Input: part model. Units: mm. Frame: model coordinates. A direction names the side the tool comes from. Coordinates: 2 decimals unless noted, no trailing zeros. Order: outer loops, then holes, each group sorted by start corner. A loop starts at its lowest first (then second) coordinate and runs counter-clockwise, first axis right, second up. Notation, with made-up numbers: M 86.25,63.25 L 137.25,63.25 A15 ccw 137.25,84.25 Z; hole C 66.5,-35 d6. An arc over 180 degrees is marked long. Answer in a Markdown table with one row per item.
from build123d import *

# Parameters (mm, degrees)
CROQUIS1_R              = 55
SALIENTE_EXTRUIR1_DEPTH = 5
CROQUIS2_R              = 1.75
CROQUIS2_R_2            = 32.5
CORTAR_EXTRUIR1_DEPTH   = 78.942286341


with BuildPart() as part:
    # Croquis1 → Saliente-Extruir1 (new body)
    with BuildSketch(Plane.XY):
        Circle(CROQUIS1_R)
    extrude(amount=SALIENTE_EXTRUIR1_DEPTH)

    # Croquis2 → Cortar-Extruir1 (cut, through all)
    with BuildSketch(Plane.XY.offset(5)):
        with Locations((0, 50)):
            Circle(CROQUIS2_R)
        with Locations((43.301270189, 25)):
            Circle(CROQUIS2_R)
        with Locations((43.301270189, -25)):
            Circle(CROQUIS2_R)
        with Locations((0, -50)):
            Circle(CROQUIS2_R)
        with Locations((-43.301270189, -25)):
            Circle(CROQUIS2_R)
        with Locations((-43.301270189, 25)):
            Circle(CROQUIS2_R)
        with Locations((0.001598992, 0.000923179)):
            Circle(CROQUIS2_R_2)
        Polygon((-21.158630785, 50.828665682), (-16.028328636, 36.733276371), (-11.329865532, 38.443377087), (-16.460167682, 52.538766399), align=None)
        Polygon((16.028328636, 36.733276371), (11.329865532, 38.443377087), (16.460167682, 52.538766399), (21.158630785, 50.828665682), align=None)
        Polygon((54.598231114, -7.090421072), (39.826114819, -4.485698407), (38.957873931, -9.409737172), (53.729990226, -12.014459837), align=None)
        Polygon((27.628008399, -29.033639916), (37.269822544, -40.524306562), (33.439600329, -43.738244611), (23.797786183, -32.247577964), align=None)
        Polygon((-33.439600329, -43.738244611), (-23.797786183, -32.247577964), (-27.628008399, -29.033639916), (-37.269822544, -40.524306562), align=None)
        Polygon((-38.957873931, -9.409737172), (-53.729990226, -12.014459837), (-54.598231114, -7.090421072), (-39.826114819, -4.485698407), align=None)
    extrude(amount=-CORTAR_EXTRUIR1_DEPTH, mode=Mode.SUBTRACT)


solid = part.part
1) Cut plane D-D, the plane y = 42. Output: boundary loops of the cut face in (x, z).
Resolved:
| item | result |
|---|---|
| outline | M -35.51,0 L -17.95,0 L -17.95,5 L -35.51,5 Z; M -12.62,0 L 12.62,0 L 12.62,5 L -12.62,5 Z; M 17.95,0 L 35.51,0 L 35.51,5 L 17.95,5 Z |
2) Material intervals for probe 1 along Y at (x, z) = (0, 3.3); probe 2 along Y at (x, z) = (-27, 4); probe 3 along X at (y, z) = (43, 2.05), sorted ascending.
Resolved:
| item | result |
|---|---|
| probe 1 | y = -55 to -51.75, -48.25 to -32.5, 32.5 to 48.25, 51.75 to 55 |
| probe 2 | y = -47.92 to -36.06, -29.56 to -18.09, 18.09 to 47.92 |
| probe 3 | x = -34.29 to -18.31, -12.99 to 12.99, 18.31 to 34.29 |
3) Contact query for flat-ended pins moving along their axis: pin 1 (1.5 mm diameter, centred on x = -23, z = 3, fed in from +Y); pin 2 (2 mm diameter, centred on x = 0, y = 50, fed in from +Z). Output: stop coordinate, or through.
Resolved:
| item | result |
|---|---|
| pin 1 | stops at y = 50.3 |
| pin 2 | passes through |
4) Cut plane A-A, the plane x = 0. Output: boundary loops of the cut face in (y, z).
Resolved:
| item | result |
|---|---|
| outline | M -55,0 L -51.75,0 L -51.75,5 L -55,5 Z; M -48.25,0 L -32.5,0 L -32.5,5 L -48.25,5 Z; M 32.5,0 L 48.25,0 L 48.25,5 L 32.5,5 Z; M 51.75,0 L 55,0 L 55,5 L 51.75,5 Z |
5) Cut plane C-C, the plane z = 2.05. State how many separate pieces and enclosed holes the cut face has, and give its area (3 significant figures).
Resolved:
| item | result |
|---|---|
| separate pieces | 1 |
| enclosed holes | 7 |
| area | 5,680 mm2 |
6) Cut plane B-B, the plane y = 29. Output: boundary loops of the cut face in (x, z), and give its area (3 significant figures).
Resolved:
| item | result |
|---|---|
| outline | M -46.73,0 L -14.67,0 L -14.67,5 L -46.73,5 Z; M 14.67,0 L 46.73,0 L 46.73,5 L 14.67,5 Z |
| area | 321 mm2 |
7) Mould query, pull axis X, two halves, no side actions, for faces 1 (the face through (24, -24, 5)), 2 (the face through (-47.748, -27.297, 2.465)), 3 (the face through (0, 55, 2)), 4 (the face through (28.668, -38.051, 2.535)). Classes: +X half, -X half, draft (parallel to the pull), parting line (faces both ways), or undercut.
Resolved:
| item | result |
|---|---|
| face 1 | draft |
| face 2 | -X half |
| face 3 | parting line |
| face 4 | undercut |
8) Reachability of faces 5 (the face through (-46.21, -10.69, 2.54)), 6 (the face through (-13.85, 45.37, 2.54)) from +Z, -Z, +X, -X, +Y, -Y: full face, straight path, thin tool, end or side. Return the list, or none.
Resolved:
| item | result |
|---|---|
| face 5 | +Z, -Z, -X |
| face 6 | +Z, -Z |
